Check sheet for the modelled part. Datum: model origin and axes. Units: mm. A direction names the side the tool comes from. Round coordinates to 2 decimals unless told otherwise and drop trailing zeros. Loops run counter-clockwise (first coordinate to the right, second up) from the corner with the lowest first, then second, coordinate; pieces in that order, holes last. Notation, with made-up numbers: M 22.5,64 L 27.5,64 A26 ccw 27.5,79 Z; hole C 34.25,21.25 d8. An arc over 180 degrees is marked long. One line per question, with ' | ' between items. Start each with the question number.
(1) Go/stop test with flat-tipped pins: P1, Ø4, axis at x = -10.5, y = 1.5, coming from the -Z side; P2, Ø5, axis at x = -20.5, z = 5.5, coming from the +Y side. Record where each tip stops, or that it passes through.
(2) Section check D-D (z = 13.5). Record the boundary of the cut face in (x, y), and give its area (3 significant figures).
(3) Section check C-C (y = 7). Record the boundary of the cut face in (x, z).
(4) Tool access check on faces 5 (the face through (-19, 0, 8)), 6 (the face through (-12.25, 14, 8)). Record the directions out of +Z, -Z, +X, -X, +Y, -Y that give a thin tool (end or side, any length) a straight path to the whole face; none if there is none.
(5) Section check A-A (x = -31). Record the boundary of the cut face in (y, z).
(6) Thickness scan on probe 1 along X at (y, z) = (12.5, 4.5); probe 2 along Z at (x, y) = (-31, 15.75); probe 3 along X at (y, z) = (12.75, 6.75). Record the ranges inside material, lowest first. Write a range as [from, to].
(7) Draft check along X on faces 1 (the face through (-24.75, 14, 8)), 2 (the face through (-7, 17, 6)), 3 (the face through (-28.8, 8.6, 8.6)), 4 (the face through (-37, 10, 8)). Enter one of: +X half, -X half, draft (parallel to the pull), parting line (faces both ways), or undercut.
(8) Section check B-B (z = 8). Record the boundary of the cut face in (x, y), and give its area (3 significant figures).
```python
from build123d import *

# Parameters (mm, degrees)
F1_DEPTH = 17
F3_D     = 4.4
F4_R     = 3


with BuildPart() as f1:
    # F0 (on Top) → F1 (new body)
    with BuildSketch(Plane.XY):
        with BuildLine():
            Line((-37, 0), (0, 0))
            Line((0, 0), (0, 17))
            Line((0, 17), (-12.25, 17))
            Line((-12.25, 17), (-12.25, 11.75))
            ThreePointArc((-12.25, 11.75), (-18.5, 5.5), (-24.75, 11.75))
            Line((-24.75, 11.75), (-24.75, 17))
            Line((-24.75, 17), (-37, 17))
            Line((-37, 17), (-37, 0))
        make_face()
    extrude(amount=F1_DEPTH)

    # F3 (through all)
    with Locations(Plane.XZ):
        with Locations((-31, 8.5445777363), (-6, 8.5445777363)):
            Hole(F3_D / 2)

    # F4
    f4_edges = [f1.edges().sort_by_distance(p)[0] for p in [
        (-37, 0, 8.5),
        (0, 0, 8.5),
        (-18.5, 0, 17),
        (-18.5, 0, 0),
        (0, 8.5, 17),
        (0, 8.5, 0),
        (-37, 8.5, 17),
        (-37, 8.5, 0),
    ]]
    fillet(f4_edges, radius=F4_R)


solid = f1.part
```
The answers:
1) P1: z = 0 | P2: y = 7.41
2) outline: M -37,3 A3 ccw -34,0 L -3,0 A3 ccw 0,3 L 0,17 L -12.25,17 L -12.25,11.75 A6.25 cw -24.75,11.75 L -24.75,17 L -37,17 Z | area: 498 mm²
3) outline: M -37,3 A3 ccw -34,0 L -22.56,0 L -22.56,17 L -34,17 A3 ccw -37,14 Z; M -14.44,0 L -3,0 A3 ccw 0,3 L 0,14 A3 ccw -3,17 L -14.44,17 Z; hole C -31,8.54 d4.4; hole C -6,8.54 d4.4
4) face 5: +Z, -Z, +X, -X, -Y | face 6: +Z, -Z, +Y
5) outline: M 0,3 A3 ccw 3,0 L 17,0 L 17,6.34 L 0,6.34 Z; M 0,10.74 L 17,10.74 L 17,17 L 3,17 A3 ccw 0,14 Z
6) probe 1: [-37, -24.75], [-12.25, 0] | probe 2: [0, 6.34], [10.74, 17] | probe 3: [-37, -32.27], [-29.73, -24.75], [-12.25, -7.27], [-4.73, 0]
7) face 1: undercut | face 2: draft | face 3: undercut | face 4: -X half
8) outline: M -37,3 A3 ccw -34,0 L -33.13,0 L -33.13,17 L -37,17 Z; M -28.87,0 L -8.13,0 L -8.13,17 L -12.25,17 L -12.25,11.75 A6.25 cw -24.75,11.75 L -24.75,17 L -28.87,17 Z; M -3.87,0 L -3,0 A3 ccw 0,3 L 0,17 L -3.87,17 Z | area: 353 mm²
